```python
from build123d import *

# Parameters (mm, degrees)
F1_W     = 77.066931
F1_H     = 56.692917
F2_DEPTH = 1
F0_R     = 0.5
F3_DEPTH = 100
F5_ANGLE = 180


with BuildPart() as f2:
    # F1 (on Top) → F2 (new body)
    with BuildSketch(Plane.XY):
        with Locations((-0.177166, -0.088582)):
            Rectangle(F1_W, F1_H)
    extrude(amount=F2_DEPTH)

    # F0 (on Top) → F3 (join)
    with BuildSketch(Plane.XY):
        with Locations((-18.665, -0.385)):
            Circle(F0_R)
        with Locations((-17.975, 9.7)):
            Circle(F0_R)
        with Locations((-19.885, 2.35)):
            Circle(F0_R)
        with Locations((-23.55, 7.2)):
            Circle(F0_R)
        with Locations((-19.875, 7.325)):
            Circle(F0_R)
        with Locations((-18.985, 18.95)):
            Circle(F0_R)
        with Locations((-26.605, 18.95)):
            Circle(F0_R)
        with Locations((-21.525, 18.95)):
            Circle(F0_R)
        with Locations((-29.145, 18.95)):
            Circle(F0_R)
        with Locations((-24.065, 18.95)):
            Circle(F0_R)
        with Locations((-18.1, 16.475)):
            Circle(F0_R)
        with Locations((-4.325, -17.525)):
            Circle(F0_R)
        with Locations((-6.825, -18.475)):
            Circle(F0_R)
        with Locations((-24.6, 14.775)):
            Circle(F0_R)
        with Locations((29.525, 16.41)):
            Circle(F0_R)
        with Locations((29.525, 13.87)):
            Circle(F0_R)
        with Locations((-21.2, 13.95)):
            Circle(F0_R)
        with Locations((29.525, 6.25)):
            Circle(F0_R)
        with Locations((-29.225, -2.075)):
            Circle(F0_R)
        with Locations((-16.325, -18.725)):
            Circle(F0_R)
        with Locations((3.45, 7.625)):
            Circle(F0_R)
        with Locations((-6.825, -20.75)):
            Circle(F0_R)
        with Locations((-29.275, -7.75)):
            Circle(F0_R)
        with Locations((-11.35, -13.05)):
            Circle(F0_R)
        with Locations((18, 17)):
            Circle(F0_R)
        with Locations((25.05, 15)):
            Circle(F0_R)
        with Locations((20.725, 16.75)):
            Circle(F0_R)
        with Locations((19, 15)):
            Circle(F0_R)
        with Locations((13.475, -8.45)):
            Circle(F0_R)
        with Locations((10.101, -8.45)):
            Circle(F0_R)
        with Locations((11.3, -6.175)):
            Circle(F0_R)
        with Locations((7.775, -12.275)):
            Circle(F0_R)
        with Locations((8.325, 11.425)):
            Circle(F0_R)
        with Locations((8.575, 8.725)):
            Circle(F0_R)
        with Locations((13.9, 15.7)):
            Circle(F0_R)
        with Locations((12.725, 7.175)):
            Circle(F0_R)
        with Locations((14.225, -5.625)):
            Circle(F0_R)
        with Locations((21.655, 18.95)):
            Circle(F0_R)
        with Locations((26.735, 18.95)):
            Circle(F0_R)
        with Locations((19.115, 18.95)):
            Circle(F0_R)
        with Locations((24.195, 18.95)):
            Circle(F0_R)
        with Locations((29.275, 18.95)):
            Circle(F0_R)
        with Locations((20.975, 13.197)):
            Circle(F0_R)
        with Locations((-29.34, 12.18)):
            Circle(F0_R)
        with Locations((29.525, 11.33)):
            Circle(F0_R)
        with Locations((-29.34, 14.72)):
            Circle(F0_R)
        with Locations((29.525, 8.79)):
            Circle(F0_R)
        with Locations((-1.5, 8)):
            Circle(F0_R)
        with Locations((-1, 14.1)):
            Circle(F0_R)
        with Locations((-7.825, -6.5)):
            Circle(F0_R)
        with Locations((-28.44, 7.2)):
            Circle(F0_R)
        with Locations((26.75, 6.35)):
            Circle(F0_R)
        with Locations((19.15, 4.55)):
            Circle(F0_R)
        with Locations((12.375, -14.2)):
            Circle(F0_R)
        with Locations((29.425, -15.2)):
            Circle(F0_R)
        with Locations((28.625, -20.975)):
            Circle(F0_R)
        with Locations((17.625, -20.575)):
            Circle(F0_R)
        with Locations((13.025, -20.474)):
            Circle(F0_R)
        with Locations((-13.375, 5.425)):
            Circle(F0_R)
        with Locations((-20.2, -20.175)):
            Circle(F0_R)
        with Locations((25.2, -5.975)):
            Circle(F0_R)
        with Locations((22.66, -5.975)):
            Circle(F0_R)
        with Locations((19.15, 0.025)):
            Circle(F0_R)
        with Locations((14.5, -12.95)):
            Circle(F0_R)
        with Locations((7.325, -8.675)):
            Circle(F0_R)
        with Locations((-12.7, 10.85)):
            Circle(F0_R)
        with Locations((-12.7, 8.4)):
            Circle(F0_R)
        with Locations((-17.825, 4.975)):
            Circle(F0_R)
        with Locations((-16.4, -15.175)):
            Circle(F0_R)
    extrude(amount=-F3_DEPTH)


with BuildPart() as f2_1:
    # F5: moved
    add(f2.part.rotate(Axis((0, 0.08858, 0), (0, -1, 0)), F5_ANGLE))


solid = f2_1.part
```
The listing builds one solid part. Answer for the finished solid, in the listing's coordinates (mm). A direction names the side the tool comes from. Give positions to 0.01 mm unless a question says otherwise; leave off trailing zeros. Order: outer loops, then holes, each group sorted by start corner. A loop starts at its lowest first (then second) coordinate and runs counter-clockwise, first axis right, second up.
Item 1: Which of the six approach directions +Z, -Z, +X, -X, +Y, -Y give full straight-line access (tool end or side, diameter ignored) to faces 1 (the face through (1, 0, -1)), 2 (the face through (1, 0, 0))?
From the geometry:
face 1: -Z, +X, -X, +Y, -Y
face 2: +Z
Item 2: Given pin 1 Ø1.5 at (x, z) = (-12, 71) entering from -Y; pin 2 Ø1 at (x, z) = (8.5, 89.5) entering from -Y; pin 3 Ø2 at (x, y) = (-28.5, -13) entering from +Z; pin 4 Ø1.5 at (y, z) = (-10, 66) entering from +X, each flat-ended and moving along its own axis, determine where each tip first touches the part or whether it passes through.
From the geometry:
pin 1: stops at y = -20.89
pin 2: stops at y = -6.97
pin 3: stops at z = 0
pin 4: passes through
Item 3: Find the intervals of material crossed by probe 1 along X at (y, z) = (-8.5, 87); probe 2 along Z at (x, y) = (7, 1.5); probe 3 along Y at (x, z) = (24.5, 59), in increasing order.
From the geometry:
probe 1: x = -13.97 to -12.98, -10.6 to -9.6, -7.79 to -6.86
probe 2: z = -1 to 0
probe 3: y = 14.29 to 15.26, 18.7 to 19.2
Item 4: The part is cut by section A-A, the plane z = 22. Count the separate pieces of the cut face and the enclosed holes in it, and give its area (3 significant figures).
From the geometry:
separate pieces: 69
enclosed holes: 0
area: 54.2 mm2
Item 5: The part is cut by section C-C, the plane y = -25. Give the vertices of the cut face in (x, z).
From the geometry:
outline: (-38.36, -1) - (38.71, -1) - (38.71, 0) - (-38.36, 0) - close
Item 6: The part is cut by section B-B, the plane x = -1. Give the vertices of the cut face in (y, z), and give its area (3 significant figures).
From the geometry:
outline: (-28.44, -1) - (28.26, -1) - (28.26, 0) - (-28.44, 0) - close
area: 56.7 mm2
